Part model, mm, in its own coordinate system. A direction names the side the tool comes from. Coordinates: 2 decimals unless noted, no trailing zeros. Write each loop counter-clockwise with the first axis right and the second up, starting at its lowest first coordinate (ties: lowest second). Pieces come first, ordered by that corner, then holes. Notation, with made-up numbers: (-33, 13) -> (6, 13) arc R28 ccw to (6, 46) -> close; hole circle Ø8 at (61.25, 41.5). An arc over 180 degrees is marked (long way). One line per question, with ' | ' between items. Start each with the question number.
Item 1: Two-plate mould, pull along Y, no slides. Class faces 4 (the flat face through (24, -13, -50)), 5 (the flat face through (37, 0, -46)), 6 (the cylindrical face through (27.1, 10.66, -2.46)): pulls with the +Y half, pulls with the -Y half, needs draft (parallel to the pull), parting line crosses it, or undercut.
Item 2: Saw through at D-D (y = 9). List the corners of the cut face in (x, z), and give its area (3 significant figures).
Item 3: Saw through at C-C (y = -1.5). List the corners of the cut face in (x, z).
Item 4: 3-axis set-ups, long thin cutter, end or side, ignore diameter. For faces 1 (the cylindrical face through (1.141, 0.28, -1.203)), 2 (the cylindrical face through (4.43, 10.14, -49.4)), 3 (the cylindrical face through (43.797, -8.619, -43.859)): which of +Z, -Z, +X, -X, +Y, -Y reach the whole face in a straight line?
Item 5: Saw through at B-B (x = 25). List the corners of the cut face in (y, z), and give its area (3 significant figures).
Item 6: Pin check, flat tips, straight feed: pin 1 (1 mm diameter, centred on x = 15, z = -13, fed in from +Y); pin 2 (18.5 mm diameter, centred on y = 3, z = -26.5, fed in from +X); pin 3 (10 mm diameter, centred on x = 41, z = -45, fed in from +Y); pin 4 (3 mm diameter, centred on x = 41.5, y = 10.5, fed in from -Z). Stop position of each tip, or through.
Item 7: Saw through at A-A (z = -35). List the corners of the cut face in (x, y).
Item 8: Probe probe 1 along Z at (x, y) = (30, -15); probe 2 along Y at (x, z) = (2, -35); probe 3 along X at (y, z) = (-13.5, -22). List the from-to ranges inside material, lowest first. Write a range as [from, to].
from build123d import *

# Parameters (mm, degrees)
EXTRUDE_1_DEPTH     = 20
CUT_EXTRUDE_2_REACH = 75.485
SKETCH_4_R          = 2.2
CUT_EXTRUDE_3_REACH = 75.485
SKETCH_5_R          = 2.2
SKETCH_3_W          = 50
SKETCH_3_H          = 50
EXTRUDE_2_DEPTH     = 20
SKETCH_10_W         = 40
SKETCH_10_H         = 40
CUT_EXTRUDE_5_DEPTH = 17
SKETCH_6_R          = 2
CUT_EXTRUDE_4_DEPTH = 37
FILLET_1_R          = 4
FILLET_2_R          = 2


with BuildPart() as part:
    # ｽｹｯﾁ1 → ﾎﾞｽ - 押し出し1 (new body)
    with BuildSketch(Plane(origin=(0, 0, 0), x_dir=(1, 0, 0), z_dir=(0, 1, 0))):
        Polygon((0, 0), (50, 0), (50, 5), (5, 5), (5, 50), (0, 50), align=None)
    extrude(amount=EXTRUDE_1_DEPTH)

    # ｽｹｯﾁ4 → ｶｯﾄ - 押し出し2 (cut, up to next)
    with BuildSketch(Plane.ZY, mode=Mode.PRIVATE) as cut_extrude_2_sk1:
        with Locations((-35, 10)):
            Circle(SKETCH_4_R)
    cut_extrude_2_tool1 = extrude(cut_extrude_2_sk1.sketch, amount=-CUT_EXTRUDE_2_REACH, mode=Mode.PRIVATE) & part.part
    add(cut_extrude_2_tool1.solids().sort_by_distance((0, 10, -35))[0], mode=Mode.SUBTRACT)

    # ｽｹｯﾁ5 → ｶｯﾄ - 押し出し3 (cut, up to next)
    with BuildSketch(Plane.XY, mode=Mode.PRIVATE) as cut_extrude_3_sk1:
        with Locations((25, 10)):
            Circle(SKETCH_5_R)
    cut_extrude_3_tool1 = extrude(cut_extrude_3_sk1.sketch, amount=-CUT_EXTRUDE_3_REACH, mode=Mode.PRIVATE) & part.part
    add(cut_extrude_3_tool1.solids().sort_by_distance((25, 10, 0))[0], mode=Mode.SUBTRACT)

    # ｽｹｯﾁ3 → ﾎﾞｽ - 押し出し2 (add)
    with BuildSketch(Plane.XZ):
        with Locations((25, -25)):
            Rectangle(SKETCH_3_W, SKETCH_3_H)
    extrude(amount=EXTRUDE_2_DEPTH)

    # ｽｹｯﾁ10 → ｶｯﾄ - 押し出し5 (cut)
    with BuildSketch(Plane(origin=(0, 0, 0), x_dir=(1, 0, 0), z_dir=(0, 1, 0))):
        with Locations((25, 25)):
            Rectangle(SKETCH_10_W, SKETCH_10_H)
    extrude(amount=-CUT_EXTRUDE_5_DEPTH, mode=Mode.SUBTRACT)

    # ｽｹｯﾁ6 → ｶｯﾄ - 押し出し4 (cut)
    with BuildSketch(Plane(origin=(0, 20, 0), x_dir=(1, 0, 0), z_dir=(0, 1, 0))):
        with Locations((5, 5)):
            Circle(SKETCH_6_R)
    extrude(amount=-CUT_EXTRUDE_4_DEPTH, mode=Mode.SUBTRACT)

    # ﾌｨﾚｯﾄ1
    fillet_1_edges = [part.edges().sort_by_distance(p)[0] for p in [
        (0, 0, 0),
        (50, -10, -50),
        (45, -8.5, -5),
        (45, -8.5, -45),
        (5, -8.5, -45),
    ]]
    fillet(fillet_1_edges, radius=FILLET_1_R)

    # ﾌｨﾚｯﾄ2
    fillet_2_edges = [part.edges().sort_by_distance(p)[0] for p in [
        (0, 0, -50),
        (5, 10, -50),
        (50, 10, -5),
        (50, 0, 0),
        (7, 1.5, -5),
        (5, 1.5, -7),
    ]]
    fillet(fillet_2_edges, radius=FILLET_2_R)


solid = part.part
From the geometry:
1) face 4: needs draft | face 5: pulls with the +Y half | face 6: undercut
2) outline: (0, -48) arc R2 ccw to (2, -50) -> (3, -50) arc R2 ccw to (5, -48) -> (5, -36.96) -> (0, -36.96) -> close; (0, -33.04) -> (5, -33.04) -> (5, -8.46) arc R2 ccw to (4, -6.73) arc R2 cw (long way) to (6.73, -4) arc R2 ccw to (8.46, -5) -> (23.04, -5) -> (23.04, 0) -> (4, 0) arc R4 ccw to (0, -4) -> close; (26.96, -5) -> (48, -5) arc R2 ccw to (50, -3) -> (50, -2) arc R2 ccw to (48, 0) -> (26.96, 0) -> close | area: 419 mm2
3) outline: (0, -48) arc R2 ccw to (2, -50) -> (46, -50) arc R4 ccw to (50, -46) -> (50, -2) arc R2 ccw to (48, 0) -> (4, 0) arc R4 ccw to (0, -4) -> close; hole (4, -6.73) arc R2 cw to (5, -8.46) -> (5, -41) arc R4 ccw to (9, -45) -> (41, -45) arc R4 ccw to (45, -41) -> (45, -9) arc R4 ccw to (41, -5) -> (8.46, -5) arc R2 cw to (6.73, -4) arc R2 ccw (long way) to start
4) face 1: +Z, -X, +Y, -Y | face 2: -Z, +X, +Y | face 3: +Y
5) outline: (-20, -50) -> (0, -50) -> (0, -45) -> (-17, -45) -> (-17, -5) -> (7.8, -5) -> (7.8, 0) -> (-20, 0) -> close; (12.2, -5) -> (20, -5) -> (20, 0) -> (12.2, 0) -> close | area: 398 mm2
6) pin 1: y = -17 | pin 2: x = 50 | pin 3: y = 0 | pin 4: z = -5
7) outline: (0, -20) -> (50, -20) -> (50, 0) -> (45, 0) -> (45, -17) -> (5, -17) -> (5, 7.8) -> (0, 7.8) -> close; (0, 12.2) -> (5, 12.2) -> (5, 20) -> (0, 20) -> close
8) probe 1: [-50, -45], [-5, 0] | probe 2: [-20, 7.8], [12.2, 20] | probe 3: [0, 5], [45, 50]
